Source: CAD feature listing. Evaluate the final solid. Frame: model axes, mm. A direction names the side the tool comes from. Round coordinates to 2 decimals unless told otherwise and drop trailing zeros. Write each loop counter-clockwise with the first axis right and the second up, starting at its lowest first coordinate (ties: lowest second). Pieces come first, ordered by that corner, then holes. Notation, with made-up numbers: M 88,-24.5 L 123,-24.5 A16 cw 123,-9.5 Z; hole C 31,-36 d6. An arc over 180 degrees is marked long. Answer in a Markdown table with one row per item.
from build123d import *

# Parameters (mm, degrees)
F0_W     = 156.015798
F0_H     = 83.234488
F1_DEPTH = 31.623
F3_DEPTH = 11.176
F4_R     = 15.516402
F5_DEPTH = 123.444


with BuildPart() as f1:
    # F0 (on Top) → F1 (new body, symmetric)
    with BuildSketch(Plane.XY):
        Rectangle(F0_W, F0_H)
    extrude(amount=F1_DEPTH, both=True)

    # F2 (on face) → F3 (join)
    with BuildSketch(Plane.XY.offset(31.623)):
        with BuildLine():
            add(Edge.make_bspline(
                [(42.055041, -8.328438), (49.456989, 29.048226), (-17.326546, 22.852551), (-84.110081, 16.656876), (-24.728494, -14.524113), (34.653093, -45.705102), (42.055041, -8.328438)],
                knots=[0, 0, 0, 2.094395, 2.094395, 4.18879, 4.18879, 6.283185, 6.283185, 6.283185], degree=2, weights=[1, 0.5, 1, 0.5, 1, 0.5, 1]))
        make_face()
    extrude(amount=F3_DEPTH)

    # F4 (on face) → F5 (join)
    with BuildSketch(Plane.XY.offset(42.799)):
        with Locations((-4.093342, 3.676504)):
            Circle(F4_R)
    extrude(amount=F5_DEPTH)


solid = f1.part
Q1. Section B-B (y = 35). Return loops of the section in (x, z).
Solutions:
| item | result |
|---|---|
| outline | M -78.01,-31.62 L 78.01,-31.62 L 78.01,31.62 L -78.01,31.62 Z |
Q2. Contact query for flat-ended pins moving along their axis: pin 1 Ø10 at (x, y) = (12.5, 26) entering from +Z; pin 2 Ø1 at (y, z) = (7, 130.5) entering from +X; pin 3 Ø4 at (x, y) = (-34.5, 14.5) entering from +Z. Output: stop coordinate, or through.
Solutions:
| item | result |
|---|---|
| pin 1 | stops at z = 31.62 |
| pin 2 | stops at x = 11.16 |
| pin 3 | stops at z = 42.8 |
Q3. Pull-direction query (X, two-part tool) for faces 3 (the flat face through (-78.008, -1, 0)), 4 (the cylindrical face through (10.707, 8.337, 103.657)), 5 (the flat face through (-1, 41.617, 0)); classes: pulls with the +X half, pulls with the -X half, needs draft (parallel to the pull), parting line crosses it, or undercut.
Solutions:
| item | result |
|---|---|
| face 3 | pulls with the -X half |
| face 4 | parting line crosses it |
| face 5 | needs draft |
Q4. Section A-A (x = 56). Return loops of the section in (y, z), and give its area (3 significant figures).
Solutions:
| item | result |
|---|---|
| outline | M -41.62,-31.62 L 41.62,-31.62 L 41.62,31.62 L -41.62,31.62 Z |
| area | 5,260 mm2 |
Q5. Access query for faces 1 (the flat face through (-1, 1, -31.623)), 2 (the flat face through (-22, -21, 31.623)). Directions: +Z, -Z, +X, -X, +Y, -Y. A direction counts if a zero-diameter tool reaches every point of the face in a straight line with its end or side. Return the directions, or none.
Solutions:
| item | result |
|---|---|
| face 1 | -Z, +X, -X, +Y, -Y |
| face 2 | +Z |
Q6. Material intervals for probe 1 along X at (y, z) = (4, 133); probe 2 along Z at (x, y) = (-28, -13); probe 3 along Z at (x, y) = (11, -2), sorted ascending.
Solutions:
| item | result |
|---|---|
| probe 1 | x = -19.61 to 11.42 |
| probe 2 | z = -31.62 to 31.62 |
| probe 3 | z = -31.62 to 42.8 |
Q7. Section C-C (z = 82). Return loops of the section in (x, y), and give its area (3 significant figures).
Solutions:
| item | result |
|---|---|
| outline | C -4.09,3.68 d31.03 |
| area | 756 mm2 |
